Check sheet for the modelled part. Datum: model origin and axes. Units: mm. A direction names the side the tool comes from. Round coordinates to 2 decimals unless told otherwise and drop trailing zeros. Loops run counter-clockwise (first coordinate to the right, second up) from the corner with the lowest first, then second, coordinate; pieces in that order, holes last. Notation, with made-up numbers: M 55.5,-9 L 63.5,-9 A27 cw 63.5,12 Z; hole C 43,60.25 d3. An arc over 180 degrees is marked long. One line per question, with ' | ' between items. Start each with the question number.
(1) Section check B-B (x = -8). Record the boundary of the cut face in (y, z).
(2) Tool access check on faces 1 (the face through (0, 5.5, 2.5)), 2 (the face through (0, 6, 3)), 3 (the face through (2.15, 3.09, 10.57)). Record the directions out of +Z, -Z, +X, -X, +Y, -Y that give a thin tool (end or side, any length) a straight path to the whole face; none if there is none.
(3) Go/stop test with flat-tipped pins: P1, Ø1, axis at y = 3, z = -9, coming from the -X side; P2, Ø2, axis at y = 3, z = 4, coming from the -X side; P3, Ø2, axis at y = 4, z = 3, coming from the +X side. Record where each tip stops, or that it passes through.
(4) Section check A-A (z = 4). Record the boundary of the cut face in (x, y), and give its area (3 significant figures).
(5) Section check D-D (z = 10.5). Record the boundary of the cut face in (x, y), and give its area (3 significant figures).
(6) Thickness scan on probe 1 along Y at (x, z) = (0, 10.5); probe 2 along Z at (x, y) = (-0.75, 4.5); probe 3 along Z at (x, y) = (6.5, 3). Record the ranges inside material, lowest first. Write a range as [from, to].
(7) Section check C-C (z = -8). Record the boundary of the cut face in (x, y), and give its area (3 significant figures).
(8) Draft check along Z on faces 4 (the face through (0, 0, 3)), 5 (the face through (-6.132, 3.042, 6.528)), 6 (the face through (3.755, 2.958, 11.923)). Enter one of: +Z half, -Z half, draft (parallel to the pull), parting line (faces both ways), or undercut.
```python
from build123d import *

# Parameters (mm, degrees)
SKETCH1_R           = 12.5
BOSS_EXTRUDE1_DEPTH = 6
CUT_EXTRUDE1_REACH  = 20.668
CUT_EXTRUDE2_REACH  = 20.668
SKETCH3_W           = 7
SKETCH3_H           = 2.4
SKETCH4_R           = 2.15
CUT_EXTRUDE3_DEPTH  = 21.426698216
SKETCH5_R           = 2.65
CUT_EXTRUDE4_DEPTH  = 19.668154869


with BuildPart() as part:
    # Sketch1 → Boss-Extrude1 (new body)
    with BuildSketch(Plane(origin=(0, 0, 0), x_dir=(1, 0, 0), z_dir=(0, 1, 0))):
        with Locations(Location((0, 0, 0), (0, 0, 270))):
            Circle(SKETCH1_R)
    extrude(amount=BOSS_EXTRUDE1_DEPTH)

    # Sketch2 → Cut-Extrude1 (cut, up to next)
    with BuildSketch(Plane(origin=(0, 6, 0), x_dir=(1, 0, 0), z_dir=(0, 1, 0)), mode=Mode.PRIVATE) as cut_extrude1_sk1:
        with BuildLine():
            ThreePointArc((0, 3.15), (-2.98307727, 1.011805317), (-1.91637679, -2.5))
            Line((-1.91637679, -2.5), (0, -2.5))
            Line((0, -2.5), (0, 3.15))
        make_face()
    cut_extrude1_tool1 = extrude(cut_extrude1_sk1.sketch, amount=-CUT_EXTRUDE1_REACH, mode=Mode.PRIVATE) & part.part
    # Sketch2 → Cut-Extrude1 (cut, up to next)
    with BuildSketch(Plane(origin=(0, 6, 0), x_dir=(1, 0, 0), z_dir=(0, 1, 0)), mode=Mode.PRIVATE) as cut_extrude1_sk2:
        with BuildLine():
            Line((0, 3.15), (0, -2.5))
            Line((0, -2.5), (1.91637679, -2.5))
            ThreePointArc((1.91637679, -2.5), (2.824808568, -1.393899766), (3.15, 0))
            ThreePointArc((3.15, 0), (2.227386361, 2.227386361), (0, 3.15))
        make_face()
    cut_extrude1_tool2 = extrude(cut_extrude1_sk2.sketch, amount=-CUT_EXTRUDE1_REACH, mode=Mode.PRIVATE) & part.part
    # Sketch2 → Cut-Extrude1 (cut, up to next)
    with BuildSketch(Plane(origin=(0, 6, 0), x_dir=(1, 0, 0), z_dir=(0, 1, 0)), mode=Mode.PRIVATE) as cut_extrude1_sk3:
        with BuildLine():
            ThreePointArc((0, 3.15), (-2.98307727, 1.011805317), (-1.91637679, -2.5))
            Line((-1.91637679, -2.5), (0, -2.5))
            Line((0, -2.5), (0, 3.15))
        make_face()
    cut_extrude1_tool3 = extrude(cut_extrude1_sk3.sketch, amount=-CUT_EXTRUDE1_REACH, mode=Mode.PRIVATE) & part.part
    # Sketch2 → Cut-Extrude1 (cut, up to next)
    with BuildSketch(Plane(origin=(0, 6, 0), x_dir=(1, 0, 0), z_dir=(0, 1, 0)), mode=Mode.PRIVATE) as cut_extrude1_sk4:
        with BuildLine():
            Line((0, 3.15), (0, -2.5))
            Line((0, -2.5), (1.91637679, -2.5))
            ThreePointArc((1.91637679, -2.5), (2.824808568, -1.393899766), (3.15, 0))
            ThreePointArc((3.15, 0), (2.227386361, 2.227386361), (0, 3.15))
        make_face()
    cut_extrude1_tool4 = extrude(cut_extrude1_sk4.sketch, amount=-CUT_EXTRUDE1_REACH, mode=Mode.PRIVATE) & part.part
    add(cut_extrude1_tool1.solids().sort_by_distance((-1.371893, 6, -0.159189))[0], mode=Mode.SUBTRACT)
    add(cut_extrude1_tool2.solids().sort_by_distance((1.371893, 6, -0.159189))[0], mode=Mode.SUBTRACT)
    add(cut_extrude1_tool3.solids().sort_by_distance((-1.371893, 6, -0.159189))[0], mode=Mode.SUBTRACT)
    add(cut_extrude1_tool4.solids().sort_by_distance((1.371893, 6, -0.159189))[0], mode=Mode.SUBTRACT)

    # Sketch3 → Cut-Extrude2 (cut, up to next)
    with BuildSketch(Plane(origin=(0, 6, 0), x_dir=(1, 0, 0), z_dir=(0, 1, 0)), mode=Mode.PRIVATE) as cut_extrude2_sk1:
        with Locations((0, -7.5)):
            Rectangle(SKETCH3_W, SKETCH3_H)
    cut_extrude2_tool1 = extrude(cut_extrude2_sk1.sketch, amount=-CUT_EXTRUDE2_REACH, mode=Mode.PRIVATE) & part.part
    add(cut_extrude2_tool1.solids().sort_by_distance((0, 6, 7.5))[0], mode=Mode.SUBTRACT)

    # Sketch4 → Cut-Extrude3 (cut, through all)
    with BuildSketch(Plane(origin=(0, 0, 2.5), x_dir=(-1, 0, 0), z_dir=(0, 0, -1))):
        with Locations((0, 3)):
            Circle(SKETCH4_R)
    extrude(amount=-CUT_EXTRUDE3_DEPTH, mode=Mode.SUBTRACT)

    # Sketch5 → Cut-Extrude4 (cut, through all)
    with BuildSketch(Plane(origin=(0, 6, 0), x_dir=(1, 0, 0), z_dir=(0, 1, 0))):
        with Locations(Location((0, 8, 0), (0, 0, 270))):
            Circle(SKETCH5_R)
        with Locations(Location((6.92820323, -4, 0), (0, 0, 270))):
            Circle(SKETCH5_R)
        with Locations(Location((-6.92820323, -4, 0), (0, 0, 270))):
            Circle(SKETCH5_R)
    extrude(amount=-CUT_EXTRUDE4_DEPTH, mode=Mode.SUBTRACT)


solid = part.part
```
The answers:
1) outline: M 0,-9.6 L 6,-9.6 L 6,1.58 L 0,1.58 Z; M 0,6.42 L 6,6.42 L 6,9.6 L 0,9.6 Z
2) face 1: +Y, -Y | face 2: +Z, -Z, +X, -X, +Y | face 3: +Z
3) P1: x = -9.17 | P2: x = -12.13 | P3: x = 12.34
4) outline: M -11.84,0 L -9.58,0 L -9.58,6 L -11.84,6 Z; M -4.28,0 L 4.28,0 L 4.28,6 L -4.28,6 Z; M 9.58,0 L 11.84,0 L 11.84,6 L 9.58,6 Z; hole C 0,3 d4.3 | area: 64.0 mm²
5) outline: M -6.78,0 L 6.78,0 L 6.78,6 L -6.78,6 Z; hole C 0,3 d4.3 | area: 66.9 mm²
6) probe 1: [0, 0.85], [5.15, 6] | probe 2: [-12.48, -10.54], [-5.46, -3.06] | probe 3: [-10.68, 1.38], [6.62, 10.68]
7) outline: M -9.6,0 L -2.65,0 L -2.65,6 L -9.6,6 Z; M 2.65,0 L 9.6,0 L 9.6,6 L 2.65,6 Z | area: 83.5 mm²
8) face 4: draft | face 5: undercut | face 6: parting line
